Job drawing, mm, ordinate dimensions from the low corner. One solid piece. A direction names the side the tool comes from. Round coordinates to 2 decimals unless told otherwise and drop trailing zeros. Loops run counter-clockwise (first coordinate to the right, second up) from the corner with the lowest first, then second, coordinate; pieces in that order, holes last. Notation, with made-up numbers: M -18.75,45 L 31.25,45 A15 cw 31.25,74 Z; hole C -26.75,63 d1. An arc over 180 degrees is marked long. Use a Markdown table: item, result. Add a question column.
(1) Which spindle directions (+Z, -Z, +X, -X, +Y, -Y) get a long thin tool onto all of the face, cutting with end or side? Do the marked faces 1 and 2. Say none if no direction does.
(2) Band-saw the part on B-B, the plane z = 22.75. Write the cut outline in (x, y).
(3) Two-plate mould, pull along Y, no slides. Class the marked faces 3, 4, 5 and 6: released by +Y, released by -Y, zero draft, split by the parting line, or undercut.
(4) Band-saw the part on C-C, the plane y = 33. Write the cut outline in (x, z) (1 decimal).
(5) Band-saw the part on D-D, the plane x = 4. Give the number of separate pieces and of enclosed holes in the cut face, and give its area (3 significant figures).
(6) Band-saw the part on A-A, the plane y = 21. Write the cut outline in (x, z).
(7) Wall check: L1, parallel to X at y = 17, z = 25.25; L2, parallel to Y at x = 22, z = 10 (1 decimal); L3, parallel to Z at x = 16, y = 18 (1 decimal). Give the ranges that are in metal, low to high.
(8) Flat gauge pins, fed straight in: P1, Ø8, axis at x = 31, z = 6.5, coming from the -Y side; P2, Ø6, axis at x = 18.5, y = 15, coming from the +Z side; P3, Ø12, axis at x = 5.5, z = 17, coming from the +Y side. Where does each tip first touch, or does it go through?
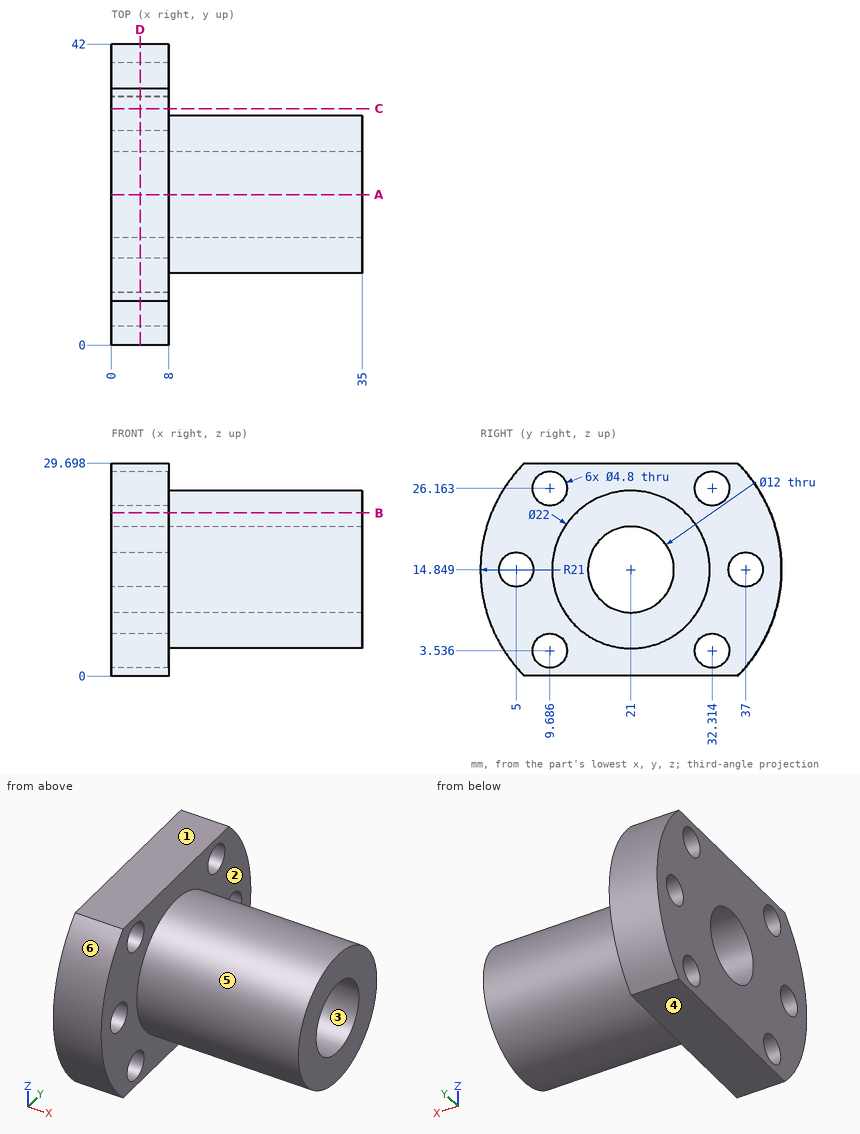
Return value:
| question | item | result |
|---|---|---|
| 1 | face 1 | +Z, +X, -X, +Y, -Y |
| 1 | face 2 | +X |
| 2 | outline | M 0,1.54 L 8,1.54 L 8,13.35 L 35,13.35 L 35,28.65 L 8,28.65 L 8,40.46 L 0,40.46 Z |
| 3 | face 3 | undercut |
| 3 | face 4 | zero draft |
| 3 | face 5 | split by the parting line |
| 3 | face 6 | released by -Y |
| 4 | outline | M 0,0 L 8,0 L 8,1.2 L 0,1.2 Z; M 0,5.8 L 8,5.8 L 8,23.9 L 0,23.9 Z; M 0,28.5 L 8,28.5 L 8,29.7 L 0,29.7 Z |
| 5 | separate pieces | 1 |
| 5 | enclosed holes | 7 |
| 5 | area | 912 mm^2 |
| 6 | outline | M 0,0 L 8,0 L 8,3.85 L 35,3.85 L 35,8.85 L 0,8.85 Z; M 0,20.85 L 35,20.85 L 35,25.85 L 8,25.85 L 8,29.7 L 0,29.7 Z |
| 7 | L1 | 0 to 8 |
| 7 | L2 | 11.1 to 17.5, 24.5 to 30.9 |
| 7 | L3 | 4.3 to 9.7, 20 to 25.4 |
| 8 | P1 | y = 10.9 |
| 8 | P2 | z = 25.43 |
| 8 | P3 | y = 42 |
